Check sheet for the modelled part. Datum: model origin and axes. Units: mm. A direction names the side the tool comes from. Give positions to 0.01 mm unless a question says otherwise; leave off trailing zeros. Order: outer loops, then holes, each group sorted by start corner. A loop starts at its lowest first (then second) coordinate and runs counter-clockwise, first axis right, second up. Notation, with made-up numbers: M 53.25,-25.75 L 66.25,-25.75 A7 cw 66.25,-21.75 Z; hole C 89.5,7 d4. An arc over 180 degrees is marked long. Answer in a Markdown table with one row per item. Add a question column.
Autodesk Inventor part; units mm, degrees
ref_plane "YZ Plane" through (0, 0, 0) normal (1, 0, 0) x (0, 1, 0)
ref_plane "XZ Plane" through (0, 0, 0) normal (0, 1, 0) x (-1, 0, 0)
ref_plane "XY Plane" through (0, 0, 0) normal (0, 0, 1) x (1, 0, 0)
sketch "Sketch1" plane through (0, 0, 0) normal (0, 0, 1) x (1, 0, 0)
  line L0 (0, 0) -> (127, 0)
  line L1 (127, 0) -> (127, 50.8)
  line L2 (127, 50.8) -> (0, 50.8)
  line L3 (0, 50.8) -> (0, 0)
  dimension "d0" = 50.8
  dimension "d1" = 127
extrude "Extrusion1" add sketch "Sketch1" along normal blind 10.16
sketch "Sketch2" plane through (0, 0, 10.16) normal (0, 0, 1) x (1, 0, 0)
  line L0 (0, 50.8) -> (0, 0)
  line L1 (127, 0) -> (127, 50.8)
  line L2 (0, 34.29) -> (127, 34.29)
  line L3 (127, 34.29) -> (127, 16.51)
  line L4 (127, 16.51) -> (0, 16.51)
  line L5 (0, 16.51) -> (0, 34.29)
  line L6 (127, 50.8) -> (0, 50.8)
  point P0 (0, 16.51)
  dimension "d4" = 17.78
  dimension "d5" = 16.51
extrude "Extrusion2" add sketch "Sketch2" along normal blind 11.43 contours L2 L1 L4 L0
sketch "Sketch4" plane through (0, 34.29, 10.16) normal (0, 1, 0) x (1, 0, 0)
  line L0 (0, 0) -> (0, -11.43)
  line L1 (127, 0) -> (127, -11.43)
  line L2 (0, -11.43) -> (127, -11.43)
  line L3 (127, -11.43) -> (127, -6.35)
  line L4 (127, -6.35) -> (0, -6.35)
  line L5 (0, -6.35) -> (0, -11.43)
  point P0 (0, 10.16)
  point P1 (0, -6.35)
  dimension "d10" = 5.08
sketch "Sketch5" plane through (0, 16.51, 10.16) normal (0, -1, 0) x (1, 0, 0)
  line L0 (0, 0) -> (0, 11.43)
  line L1 (127, 0) -> (127, 11.43)
  line L2 (0, 11.43) -> (127, 11.43)
  line L3 (127, 11.43) -> (127, 6.35)
  line L4 (127, 6.35) -> (0, 6.35)
  line L5 (0, 6.35) -> (0, 11.43)
  point P0 (0, -10.16)
  point P1 (0, 6.35)
  dimension "d11" = 5.08
extrude "Extrusion3" add sketch "Sketch5" along normal blind 6.35
extrude "Extrusion4" add sketch "Sketch4" along normal blind 6.35
sketch "Sketch6" plane through (0, 0, 0) normal (0, 0, -1) x (-1, 0, 0)
  circle A0 centre (-63.5, 25.4) radius 5.08
  line L0 (0, 50.8) -> (0, 0)
  line L1 (0, 0) -> (-127, 0)
  dimension "d16" = 10.16
  dimension "d17" = 63.5
  dimension "d18" = 25.4
hole "Hole1" at (63.5, 25.4, 0) direction (0, 0, 1) diameter 9.017 end through all
properties part number "jeep pvc connect on pvc"
Q1. Cross-section at A-A (x = 63.5). Record the boundary of the cut face in (y, z).
Q2. Cross-section at B-B (y = 12.5). Record the boundary of the cut face in (x, z), and give its area (3 significant figures).
Q3. Tool access check on faces 5 (the flat face through (63, 43, 10.16)), 6 (the flat face through (64, 13, 16.51)), 7 (the flat face through (63, 10.16, 19)), 8 (the flat face through (63, 40.64, 19)). Record the directions out of +Z, -Z, +X, -X, +Y, -Y that give a thin tool (end or side, any length) a straight path to the whole face; none if there is none.
Q4. Cross-section at C-C (z = 19). Record the boundary of the cut face in (x, y).
Q5. Thickness scan on probe 1 along X at (y, z) = (25.4, 12.25); probe 2 along Z at (x, y) = (63, 40); probe 3 along Y at (x, z) = (19, 20.75). Record the ranges inside material, lowest first.
Q6. Go/stop test with flat-tipped pins: pin 1 (12 mm diameter, centred on y = 5.5, z = 17, fed in from +X); pin 2 (5.5 mm diameter, centred on x = 81, z = 19, fed in from -Y); pin 3 (5 mm diameter, centred on x = 33, z = 13, fed in from +Y); pin 4 (4 mm diameter, centred on x = 93.5, z = 18, fed in from +Y). Record where each tip stops, or that it passes through.
Q7. Draft check along Z on faces 1 (the flat face through (63, 34.29, 13)), 2 (the flat face through (64, 16.51, 13)), 3 (the flat face through (63, 20, 0)), 4 (the cylindrical face through (67.9, 24.42, 10.95)). Enter one of: pulls with the +Z half, pulls with the -Z half, needs draft (parallel to the pull), parting line crosses it, or undercut.
Q8. Cross-section at D-D (x = 48). Record the boundary of the cut face in (y, z).
Values follow:
| question | item | result |
|---|---|---|
| 1 | outline | M 0,0 L 20.89,0 L 20.89,21.59 L 10.16,21.59 L 10.16,16.51 L 16.51,16.51 L 16.51,10.16 L 0,10.16 Z; M 29.91,0 L 50.8,0 L 50.8,10.16 L 34.29,10.16 L 34.29,16.51 L 40.64,16.51 L 40.64,21.59 L 29.91,21.59 Z |
| 2 | outline | M 0,0 L 127,0 L 127,10.16 L 0,10.16 Z; M 0,16.51 L 127,16.51 L 127,21.59 L 0,21.59 Z |
| 2 | area | 1,940 mm² |
| 3 | face 5 | +X, -X, +Y |
| 3 | face 6 | +X, -X, -Y |
| 3 | face 7 | +Z, +X, -X, -Y |
| 3 | face 8 | +Z, +X, -X, +Y |
| 4 | outline | M 0,10.16 L 127,10.16 L 127,40.64 L 0,40.64 Z; hole C 63.5,25.4 d9.02 |
| 5 | probe 1 | 0 to 58.99, 68.01 to 127 |
| 5 | probe 2 | 0 to 10.16, 16.51 to 21.59 |
| 5 | probe 3 | 10.16 to 40.64 |
| 6 | pin 1 | x = 127 |
| 6 | pin 2 | y = 10.16 |
| 6 | pin 3 | y = 34.29 |
| 6 | pin 4 | y = 40.64 |
| 7 | face 1 | undercut |
| 7 | face 2 | undercut |
| 7 | face 3 | pulls with the -Z half |
| 7 | face 4 | needs draft |
| 8 | outline | M 0,0 L 50.8,0 L 50.8,10.16 L 34.29,10.16 L 34.29,16.51 L 40.64,16.51 L 40.64,21.59 L 10.16,21.59 L 10.16,16.51 L 16.51,16.51 L 16.51,10.16 L 0,10.16 Z |
